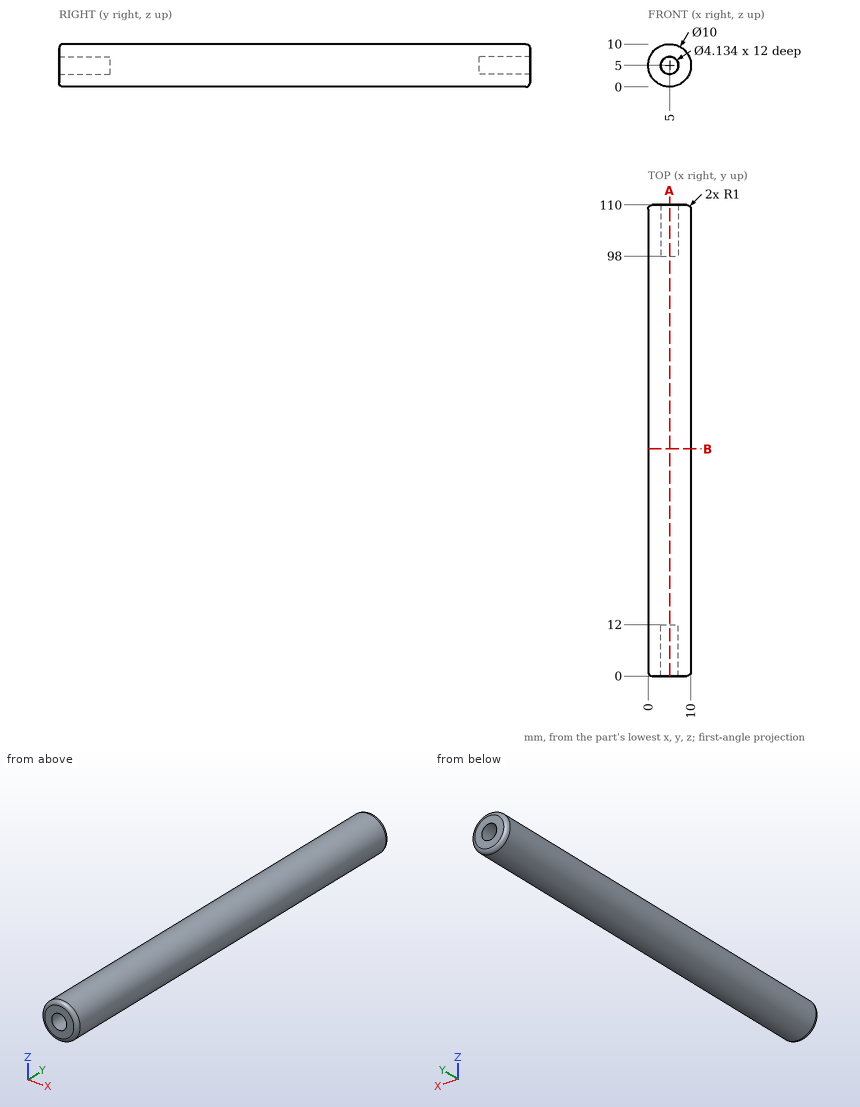
Part print with two shaded views. Sizes in mm from the minimum x, y, z corner. Round coordinates to 2 decimals unless told otherwise and drop trailing zeros. Order: outer loops, then holes, each group sorted by start corner. A loop starts at its lowest first (then second) coordinate and runs counter-clockwise, first axis right, second up.
(1) Pin check, flat tips, straight feed: pin 1 (3.5 mm diameter, centred on x = 5, z = 5, fed in from -Y); pin 2 (3.5 mm diameter, centred on x = 5, z = 5, fed in from +Y); pin 3 (1 mm diameter, centred on y = 50, z = 8.5, fed in from +X). Stop position of each tip, or through.
(2) Band-saw the part on A-A (x = 5). List the corners of the cut face in (y, z), then the cut area to 4 significant figures.
(3) Drill centre lines: line 1 (Z direction, x = 5, y = 105.5); line 2 (Z direction, x = 8, y = 29). Where is each one in solid material? Low to high.
(4) Band-saw the part on B-B (y = 53). List the corners of the cut face in (x, z).
Verdict:
1. pin 1: stops at y = 12
1. pin 2: stops at y = 98
1. pin 3: stops at x = 9
2. outline: (0, 1) arc R1 ccw to (1, 0) - (109, 0) arc R1 ccw to (110, 1) - (110, 2.93) - (98, 2.93) - (98, 7.07) - (110, 7.07) - (110, 9) arc R1 ccw to (109, 10) - (1, 10) arc R1 ccw to (0, 9) - (0, 7.07) - (12, 7.07) - (12, 2.93) - (0, 2.93) - close
2. area: 1,000 mm2
3. line 1: z = 0 to 2.93, 7.07 to 10
3. line 2: z = 1 to 9
4. outline: circle Ø10 at (5, 5)
